Print and shaded views of the part. All mm, measured from the part's lowest x, y and z. Round coordinates to 2 decimals unless told otherwise and drop trailing zeros. Write each loop counter-clockwise with the first axis right and the second up, starting at its lowest first coordinate (ties: lowest second). Pieces come first, ordered by that corner, then holes.
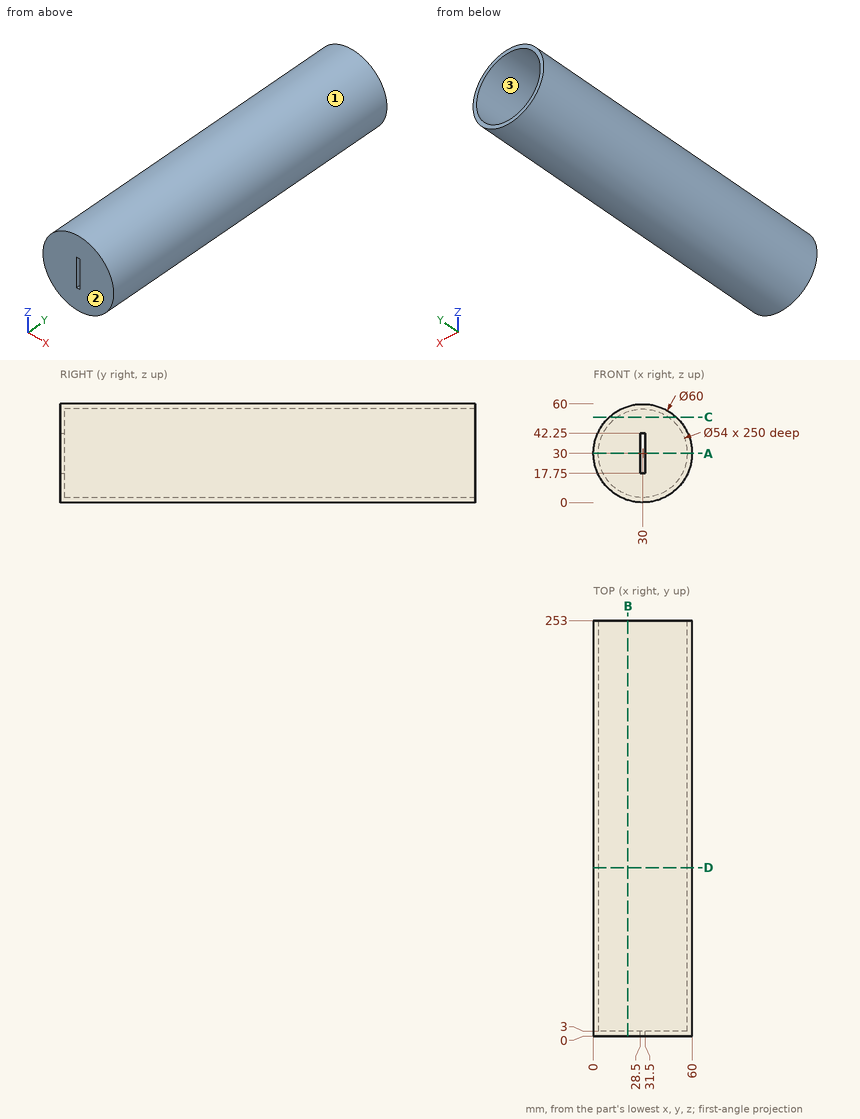
1) Mould opens along Z. For the marked faces 1, 2 and 3 say: released by +Z, released by -Z, zero draft, split by the parting line, or undercut.
Results:
face 1: split by the parting line
face 2: zero draft
face 3: undercut
2) Slice it at A-A (z = 30). Write the cut outline in (x, y).
Results:
outline: (0, 0) - (28.5, 0) - (28.5, 3) - (3, 3) - (3, 253) - (0, 253) - close; (31.5, 0) - (60, 0) - (60, 253) - (57, 253) - (57, 3) - (31.5, 3) - close
3) Wall check: L1, parallel to X at y = 186, z = 30; L2, parallel to Y at x = 19.5, z = 36.5. Give the ranges that are in metal, low to high.
Results:
L1: x = 0 to 3, 57 to 60
L2: y = 0 to 3
4) Slice it at B-B (x = 21). Write the cut outline in (y, z).
Results:
outline: (0, 1.38) - (253, 1.38) - (253, 4.54) - (3, 4.54) - (3, 55.46) - (253, 55.46) - (253, 58.62) - (0, 58.62) - close
5) Pin check, flat tips, straight feed: pin 1 Ø2.5 at (x, y) = (29.5, 2) entering from -Z; pin 2 Ø1.5 at (y, z) = (2, 25.5) entering from -X; pin 3 Ø4 at (y, z) = (139, 37) entering from +X. Stop position of each tip, or through.
Results:
pin 1: stops at z = 0
pin 2: stops at x = 0.24
pin 3: stops at x = 59.58
6) Slice it at D-D (y = 102.5). Write the cut outline in (x, z), plus the area to 3 significant figures.
Results:
outline: circle Ø60 at (30, 30); hole circle Ø54 at (30, 30)
area: 537 mm2
7) Slice it at C-C (z = 52). Write the cut outline in (x, y).
Results:
outline: (9.6, 0) - (50.4, 0) - (50.4, 253) - (45.65, 253) - (45.65, 3) - (14.35, 3) - (14.35, 253) - (9.6, 253) - close
